Build history of the part. All positions in model axes, mm. Face numbers are marked on the shaded views. A direction names the side the tool comes from. Give positions to 0.01 mm unless a question says otherwise; leave off trailing zeros. Write each loop counter-clockwise with the first axis right and the second up, starting at its lowest first coordinate (ties: lowest second). Pieces come first, ordered by that corner, then holes. Notation, with made-up numbers: M 23,-1 L 47,-1 A30 cw 47,25 Z; hole C 13.25,32 d8. An arc over 180 degrees is marked long. Return JSON: item names as keys, results as strings. Group by question number.
Q1. Tool access for the marked faces 1 and 2: list every direction of +Z, -Z, +X, -X, +Y, -Y with a clear straight run to the whole face (end or side of a thin tool).
Q2. Pull direction Y, two halves, no side cores. Call the marked faces 3, 4 and 5: +Y half, -Y half, draft (parallel to the pull), parting line (faces both ways), or undercut.
Q3. Wall check: probe 1 along Y at (x, z) = (-68, 12.25); probe 2 along Y at (x, z) = (-44, 22); probe 3 along Y at (x, z) = (-71, 24.25). Give the ranges that are in metal, low to high.
Q4. Band-saw the part on B-B, the plane z = 8.5. Count the separate pieces of the cut face and the enclosed holes in it, then the cut area to 3 significant figures.
Q5. Band-saw the part on C-C, the plane x = -67. Give the cut face in (y, z).
Q6. Flat gauge pins, fed straight in: pin 1 Ø2 at (y, z) = (55, 21.5) entering from +X; pin 2 Ø3 at (x, z) = (48.5, 7) entering from +Y; pin 3 Ø7 at (y, z) = (16.5, 17) entering from +X. Where does each tip first touch, or does it go through?
Q7. Band-saw the part on D-D, the plane x = 29. Give the cut face in (y, z), then the cut area to 3 significant figures.
Q8. Band-saw the part on A-A, the plane y = 2.5. Give the cut face in (x, z), then the cut area to 3 significant figures.
from build123d import *

# Parameters (mm, degrees)
SKETCH2_R           = 6
SKETCH2_R_2         = 15
BOSS_EXTRUDE1_DEPTH = 30


with BuildPart() as part:
    # Sketch2 → Boss-Extrude1 (new body)
    with BuildSketch(Plane.XY):
        with BuildLine():
            Line((-90.841121495, 71.557977192), (-90.841121495, -30.442022808))
            Line((-90.841121495, -30.442022808), (64.158878505, -30.442022808))
            Line((64.158878505, -30.442022808), (64.158878505, -8.442022808))
            ThreePointArc((64.158878505, -8.442022808), (61.815732754, -2.785168558), (56.158878505, -0.442022808))
            Line((56.158878505, -0.442022808), (26.60450497, -0.442022808))
            ThreePointArc((26.60450497, -0.442022808), (21.352247656, 1.523592956), (18.680970285, 6.454528916))
            ThreePointArc((18.680970285, 6.454528916), (4.514217564, 34.913316251), (-23.944569771, 49.080068973))
            ThreePointArc((-23.944569771, 49.080068973), (-28.875505731, 51.751346343), (-30.841121495, 57.003603657))
            Line((-30.841121495, 57.003603657), (-30.841121495, 71.557977192))
            ThreePointArc((-30.841121495, 71.557977192), (-33.184267246, 77.214831442), (-38.841121495, 79.557977192))
            Line((-38.841121495, 79.557977192), (-82.841121495, 79.557977192))
            ThreePointArc((-82.841121495, 79.557977192), (-88.497975745, 77.214831442), (-90.841121495, 71.557977192))
        make_face()
        with Locations((-70.841121495, -15.442022808)):
            Circle(SKETCH2_R, mode=Mode.SUBTRACT)
        with Locations((-50.841121495, -15.442022808)):
            Circle(SKETCH2_R, mode=Mode.SUBTRACT)
        with Locations((-30.841121495, -15.442022808)):
            Circle(SKETCH2_R, mode=Mode.SUBTRACT)
        with Locations((-10.841121495, -15.442022808)):
            Circle(SKETCH2_R, mode=Mode.SUBTRACT)
        with Locations((9.158878505, -15.442022808)):
            Circle(SKETCH2_R, mode=Mode.SUBTRACT)
        with Locations((29.158878505, -15.442022808)):
            Circle(SKETCH2_R, mode=Mode.SUBTRACT)
        with Locations((49.158878505, -15.442022808)):
            Circle(SKETCH2_R, mode=Mode.SUBTRACT)
        with Locations((-60.841121495, 59.557977192)):
            Circle(SKETCH2_R_2, mode=Mode.SUBTRACT)
        with BuildLine():
            Line((-62.841121495, -0.442022808), (-10.347219963, -0.442022808))
            ThreePointArc((-10.347219963, -0.442022808), (-3.741437373, 3.045368594), (-2.894892134, 10.467068101))
            ThreePointArc((-2.894892134, 10.467068101), (-13.918839251, 24.329661907), (-30.841121495, 29.557977192))
            Line((-30.841121495, 29.557977192), (-62.841121495, 29.557977192))
            ThreePointArc((-62.841121495, 29.557977192), (-68.497975745, 27.214831442), (-70.841121495, 21.557977192))
            Line((-70.841121495, 21.557977192), (-70.841121495, 7.557977192))
            ThreePointArc((-70.841121495, 7.557977192), (-68.497975745, 1.901122943), (-62.841121495, -0.442022808))
        make_face(mode=Mode.SUBTRACT)
    extrude(amount=BOSS_EXTRUDE1_DEPTH)


solid = part.part
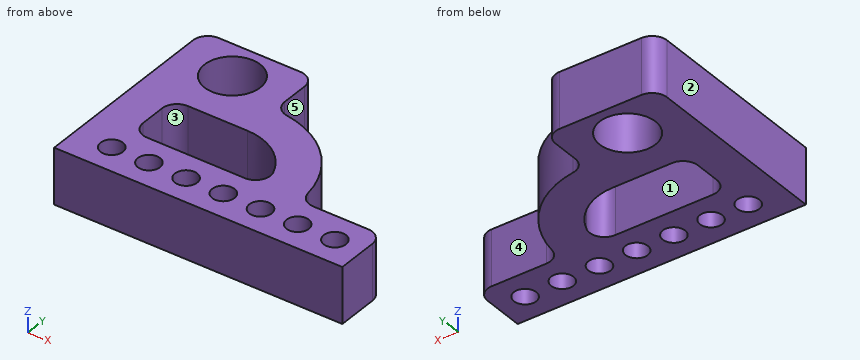
From the geometry:
{
 "1": {"face 1": "+Z, -Z", "face 2": "+Z, -Z, -X, +Y, -Y"},
 "2": {"face 3": "undercut", "face 4": "+Y half", "face 5": "draft"},
 "3": {"probe 1": "y = -30.44 to -20.73, -10.16 to 1.44, 27.67 to 46.38, 72.74 to 79.56", "probe 2": "y = -30.44 to -0.44, 29.56 to 79.56", "probe 3": "y = -30.44 to -21.44, -9.44 to 48.52, 70.59 to 79.56"},
 "4": {"separate pieces": "1", "enclosed holes": "9", "area": "8,040 mm^2"},
 "5": {"outline": "M -30.44,0 L -20.05,0 L -20.05,30 L -30.44,30 Z; M -10.83,0 L 0.72,0 L 0.72,30 L -10.83,30 Z; M 28.39,0 L 45.88,0 L 45.88,30 L 28.39,30 Z; M 73.24,0 L 79.56,0 L 79.56,30 L 73.24,30 Z"},
 "6": {"pin 1": "stops at x = -30.26", "pin 2": "stops at y = -0.44", "pin 3": "stops at x = 17.32"},
 "7": {"outline": "M -30.44,0 L -21.44,0 L -21.44,30 L -30.44,30 Z; M -9.44,0 L -0.44,0 L -0.44,30 L -9.44,30 Z", "area": "540 mm^2"},
 "8": {"outline": "M -90.84,0 L -69.04,0 L -69.04,30 L -90.84,30 Z; M -4.15,0 L 20.41,0 L 20.41,30 L -4.15,30 Z", "area": "1,390 mm^2"}
}
